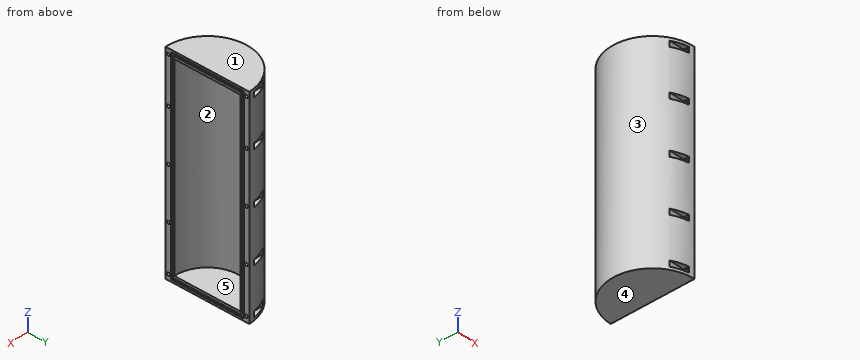
from build123d import *

# Parameters (mm, degrees)
BOSS_EXTRUDE1_DEPTH            = 280
BOSS_EXTRUDE3_START            = 10
BOSS_EXTRUDE3_DEPTH            = 10
CUT_EXTRUDE_THIN1_START        = -2
CUT_EXTRUDE_THIN1_DEPTH        = 2
FILLET6_R                      = 1
SKETCH11_W                     = 8
SKETCH11_H                     = 8
SKETCH11_W_2                   = 8.009527264
CUT_EXTRUDE1_DEPTH             = 51
M4_CLEARANCE_HOLE1_D           = 4.5
M4_CLEARANCE_HOLE1_CSINK_D     = 4.55
M4_CLEARANCE_HOLE1_CSINK_ANGLE = 90


# Read off the part's stored shape, not the designer's step: Cut-Extrude-Thin1
with BuildPart() as part:
    # Sketch1 → Boss-Extrude1 (new body)
    with BuildSketch(Plane.XY):
        with BuildLine():
            Line((0, 52), (-2, 52))
            Line((-2, 52), (-2, 48.5))
            Line((-2, 48.5), (0, 48.5))
            Line((0, 48.5), (0, 47.5))
            ThreePointArc((0, 47.5), (-47.5, 0), (0, -47.5))
            Line((0, -47.5), (0, -48.5))
            Line((0, -48.5), (-2, -48.5))
            Line((-2, -48.5), (-2, -52))
            Line((-2, -52), (0, -52))
            Line((0, -52), (0, -60))
            ThreePointArc((0, -60), (-60, 0), (0, 60))
            Line((0, 60), (0, 52))
        make_face()
    extrude(amount=-BOSS_EXTRUDE1_DEPTH)

    # Sketch7 → Boss-Extrude3 (add)
    with BuildSketch(Plane.XY.offset(BOSS_EXTRUDE3_START)):
        with BuildLine():
            Line((0, 60), (0, -60))
            ThreePointArc((0, -60), (-60, 0), (0, 60))
        make_face()
    boss_extrude3 = extrude(amount=-BOSS_EXTRUDE3_DEPTH)

    # Mirror1: Boss-Extrude3 across plane
    add(boss_extrude3.mirror(Plane.XY.offset(-140)))

    # Cut-Extrude-Thin1 outline → Cut-Extrude-Thin1 (cut)
    with BuildSketch(Plane(origin=(0, 0, 0), x_dir=(0, 0, -1), z_dir=(1, 0, 0)).offset(CUT_EXTRUDE_THIN1_START)):
        Polygon((0, 52), (-7, 52), (-7, -52), (0, -52), (0, -48.5), (-3.5, -48.5), (-3.5, 48.5), (0, 48.5), align=None)
    cut_extrude_thin1 = extrude(amount=CUT_EXTRUDE_THIN1_DEPTH, mode=Mode.SUBTRACT)

    # Mirror2: Cut-Extrude-Thin1 across plane
    add(cut_extrude_thin1.mirror(Plane.XY.offset(-140)), mode=Mode.SUBTRACT)

    # Fillet6
    fillet6_edges = [part.edges().sort_by_distance(p)[0] for p in [
        (-1, -52, 7),
        (-1, 52, 7),
        (-1, 48.5, 3.5),
        (-1, -48.5, 3.5),
        (-1, -52, -287),
        (-1, -48.5, -283.5),
        (-1, 48.5, -283.5),
        (-1, 52, -287),
    ]]
    fillet(fillet6_edges, radius=FILLET6_R)

    # Sketch11 → Cut-Extrude1 (cut)
    with BuildSketch(Plane(origin=(-59.040249017, 0, 0), x_dir=(0, 0, -1), z_dir=(-1, 0, 0))):
        with Locations((139.975606131, 56)):
            Rectangle(SKETCH11_W, SKETCH11_H)
        with Locations((-2, 56)):
            Rectangle(SKETCH11_W, SKETCH11_H)
        with Locations((-2, -55.889665958)):
            Rectangle(SKETCH11_W, SKETCH11_H)
        with Locations((139.975606131, -55.889665958)):
            Rectangle(SKETCH11_W, SKETCH11_H)
        with Locations((281.951212263, 56)):
            Rectangle(SKETCH11_W, SKETCH11_H)
        with Locations((281.951212263, -55.889665958)):
            Rectangle(SKETCH11_W, SKETCH11_H)
        with Locations((64.992566698, 56)):
            Rectangle(SKETCH11_W_2, SKETCH11_H)
        with Locations((214.958645565, 56)):
            Rectangle(SKETCH11_W_2, SKETCH11_H)
        with Locations((214.958645565, -55.889665958)):
            Rectangle(SKETCH11_W_2, SKETCH11_H)
        with Locations((64.992566698, -55.889665958)):
            Rectangle(SKETCH11_W_2, SKETCH11_H)
    extrude(amount=-CUT_EXTRUDE1_DEPTH, mode=Mode.SUBTRACT)

    # M4 Clearance Hole1 (through all)
    with Locations(Plane.ZY.offset(8.040249017)):
        with Locations((-281.951212263, 55.889665958), (-281.951212263, -56), (-139.973202333, -56), (2, -56), (2, 55.912652005), (-139.975606131, 55.912652005), (-214.982691693, 55.889665958), (-64.963712973, 55.889665958), (-214.982691693, -56), (-64.963712973, -56)):
            CounterSinkHole(M4_CLEARANCE_HOLE1_D / 2, M4_CLEARANCE_HOLE1_CSINK_D / 2, counter_sink_angle=M4_CLEARANCE_HOLE1_CSINK_ANGLE)


solid = part.part
Part model, mm, in its own coordinate system. Face numbers are marked on the shaded views. A direction names the side the tool comes from. Give positions to 0.01 mm unless a question says otherwise; leave off trailing zeros. Write each loop counter-clockwise with the first axis right and the second up, starting at its lowest first coordinate (ties: lowest second). Pieces come first, ordered by that corner, then holes.
1) Cut at A-A on z = -76. Write the cut outline in (x, y).
Resolved:
outline: (-2, -52) - (-2, -48.5) - (0, -48.5) - (0, -47.5) arc R47.5 cw to (0, 47.5) - (0, 48.5) - (-2, 48.5) - (-2, 52) - (0, 52) - (0, 60) arc R60 ccw to (0, -60) - (0, -52) - close
2) Probe L1, parallel to Z at x = -4, y = -56; L2, parallel to Z at x = -13.5, y = 37; L3, parallel to Y at x = -44, z = -58.5. List the from-to ranges inside material, lowest first.
Resolved:
L1: z = -290 to -284.2, -279.7 to -217.23, -212.73 to -142.22, -137.72 to -67.21, -62.71 to -0.25, 4.25 to 10
L2: z = -290 to -280, 0 to 10
L3: y = -40.79 to -17.9, 17.9 to 40.79
3) Cut at B-B on x = -43. Write the cut outline in (y, z), then the cut area to 3 significant figures.
Resolved:
outline: (-41.84, -290) - (41.84, -290) - (41.84, 10) - (-41.84, 10) - close; hole (-20.18, -280) - (20.18, -280) - (20.18, 0) - (-20.18, 0) - close
area: 13,800 mm2
4) Cut at C-C on y = 0. Write the cut outline in (x, z), then the cut area to 3 significant figures.
Resolved:
outline: (-60, -290) - (0, -290) - (0, -287) - (-2, -287) - (-2, -283.5) - (0, -283.5) - (0, -280) - (-47.5, -280) - (-47.5, 0) - (0, 0) - (0, 3.5) - (-2, 3.5) - (-2, 7) - (0, 7) - (0, 10) - (-60, 10) - close
area: 4,690 mm2
5) Two-plate mould, pull along Y, no slides. Class the marked faces 1, 2 and 3: released by +Y, released by -Y, zero draft, split by the parting line, or undercut.
Resolved:
face 1: zero draft
face 2: undercut
face 3: split by the parting line
6) Which spindle directions (+Z, -Z, +X, -X, +Y, -Y) get a long thin tool onto all of the face, cutting with end or side? Do the marked faces 4 and 5. Say none if no direction does.
Resolved:
face 4: -Z, +X, -X, +Y, -Y
face 5: +X
7) Pin check, flat tips, straight feed: pin 1 (8 mm diameter, centred on x = -20.5, z = -66.5, fed in from +Y); pin 2 (8 mm diameter, centred on y = -54.5, z = -139.5, fed in from -X); pin 3 (6.5 mm diameter, centred on x = -20, z = -282, fed in from -Y); pin 4 (4 mm diameter, centred on x = -19.5, y = 57, fed in from +Z). Stop position of each tip, or through.
Resolved:
pin 1: stops at y = 57.43
pin 2: stops at x = -32.4
pin 3: stops at y = -52
pin 4: stops at z = 10
